The listing builds one solid part. Answer for the finished solid, in the listing's coordinates (mm). A direction names the side the tool comes from. Round coordinates to 2 decimals unless told otherwise and drop trailing zeros. Loops run counter-clockwise (first coordinate to the right, second up) from the corner with the lowest first, then second, coordinate; pieces in that order, holes last. Notation, with made-up numbers: M 1,80.5 L 7,80.5 A13 cw 7,96.5 Z; hole C -4,61.25 d7. An arc over 180 degrees is marked long. Put each result on its own line as item: value. Start each with the question number.
(1) Determine the mould class of faces 4 (the face through (-66, 25.4, -17)), 5 (the face through (-50.651, 22.269, 85.774)), 6 (the face through (-102.283, 22.181, -22.713)) for opening direction X: released by +X, released by -X, zero draft, split by the parting line, or undercut.
(2) Section B-B, the plane z = 0 is taken. Determine the outline of the cut face in (x, y) (3 decimals).
(3) Section A-A, the plane x = 0 is taken. Determine the outline of the cut face in (y, z) (3 decimals).
(4) Which of the six approach directions +Z, -Z, +X, -X, +Y, -Y give full straight-line access (tool end or side, diameter ignored) to faces 1 (the face through (-94.7, 22.3, 0.1)), 2 (the face through (-62, 19.05, 54)), 3 (the face through (73.663, 23.434, -9.672))?
(5) Section D-D, the plane z = -64.5 is taken. Determine the outline of the cut face in (x, y), then the cut area to 3 significant figures.
(6) Flat-ended cylindrical pins translate along their axes: P1, Ø6.5, axis at x = 0, z = -97.25, coming from the -Y side; P2, Ø4, axis at x = -22.5, y = 18, coming from the -Z side; P3, Ø12, axis at x = -42.5, y = 3.5, coming from the -Z side; P4, Ø4, axis at x = 84.22, z = 48.63, coming from the -Y side. Find the tip coordinate at first contact, or state that the pin passes through.
(7) Straight lines are drawn through the part: line 1 (Z direction, x = -16, y = 23.75); line 2 (Z direction, x = 2.5, y = 6.25); line 3 (X direction, y = 4.25, z = -6). For each, find the intervals that lie inside material, in ascending order.
(8) Section C-C, the plane x = -31.5 is taken. Determine the outline of the cut face in (y, z), then the cut area to 3 significant figures.
```python
from build123d import *

# Parameters (mm, degrees)
SKETCH1_R            = 80.518
SKETCH1_R_2          = 67.818
INNER_CYLINDER_DEPTH = 19.05
SKETCH2_R            = 104.775
SKETCH2_R_2          = 67.818
FLANGE_DEPTH         = 6.35
SKETCH4_R            = 81.407
SKETCH4_R_2          = 74.295
GROOVE_DEPTH         = 3.9878
SKETCH5_R            = 2.5527
SCREW_HOLES_DEPTH    = 6.35
CIRPATTERN1_COUNT    = 12


with BuildPart() as part:
    # Sketch1 → Inner Cylinder (new body)
    with BuildSketch(Plane(origin=(0, 0, 0), x_dir=(1, 0, 0), z_dir=(0, 1, 0))):
        with Locations(Location((0, 0, 0), (0, 0, 90))):
            Circle(SKETCH1_R)
        with Locations(Location((0, 0, 0), (0, 0, 90))):
            Circle(SKETCH1_R_2, mode=Mode.SUBTRACT)
    extrude(amount=INNER_CYLINDER_DEPTH)

    # Sketch2 → Flange (add)
    with BuildSketch(Plane(origin=(0, 19.05, 0), x_dir=(1, 0, 0), z_dir=(0, 1, 0))):
        with Locations(Location((0, 0, 0), (0, 0, 270))):
            Circle(SKETCH2_R)
        with Locations(Location((0, 0, 0), (0, 0, 90))):
            Circle(SKETCH2_R_2, mode=Mode.SUBTRACT)
    extrude(amount=FLANGE_DEPTH)

    # Sketch4 → Groove (cut)
    with BuildSketch(Plane(origin=(0, 25.4, 0), x_dir=(1, 0, 0), z_dir=(0, 1, 0))):
        with Locations(Location((0, 0, 0), (0, 0, 270))):
            Circle(SKETCH4_R)
        with Locations(Location((0, 0, 0), (0, 0, 270))):
            Circle(SKETCH4_R_2, mode=Mode.SUBTRACT)
    extrude(amount=-GROOVE_DEPTH, mode=Mode.SUBTRACT)

    # Sketch5 → Screw Holes (cut)
    with BuildSketch(Plane(origin=(0, 25.4, 0), x_dir=(1, 0, 0), z_dir=(0, 1, 0))):
        with Locations(Location((0, -97.25025, 0), (0, 0, 270))):
            Circle(SKETCH5_R)
    screw_holes = extrude(amount=-SCREW_HOLES_DEPTH, mode=Mode.SUBTRACT)

    # CirPattern1: Screw Holes ×12 about axis
    cirpattern1_axis = Axis((0, 0, 0), (0, 1, 0))
    for i in range(1, CIRPATTERN1_COUNT):
        add(screw_holes.rotate(cirpattern1_axis, i * 360 / CIRPATTERN1_COUNT), mode=Mode.SUBTRACT)


solid = part.part
```
Recorded:
1. face 4: zero draft
1. face 5: undercut
1. face 6: split by the parting line
2. outline: M -104.775,19.05 L -99.803,19.05 L -99.803,25.4 L -104.775,25.4 Z; M -94.698,19.05 L -80.518,19.05 L -80.518,0 L -67.818,0 L -67.818,25.4 L -74.295,25.4 L -74.295,21.412 L -81.407,21.412 L -81.407,25.4 L -94.698,25.4 Z; M 67.818,0 L 80.518,0 L 80.518,19.05 L 94.698,19.05 L 94.698,25.4 L 81.407,25.4 L 81.407,21.412 L 74.295,21.412 L 74.295,25.4 L 67.818,25.4 Z; M 99.803,19.05 L 104.775,19.05 L 104.775,25.4 L 99.803,25.4 Z
3. outline: M 0,-80.518 L 19.05,-80.518 L 19.05,-94.698 L 25.4,-94.698 L 25.4,-81.407 L 21.412,-81.407 L 21.412,-74.295 L 25.4,-74.295 L 25.4,-67.818 L 0,-67.818 Z; M 0,67.818 L 25.4,67.818 L 25.4,74.295 L 21.412,74.295 L 21.412,81.407 L 25.4,81.407 L 25.4,94.698 L 19.05,94.698 L 19.05,80.518 L 0,80.518 Z; M 19.05,-104.775 L 25.4,-104.775 L 25.4,-99.803 L 19.05,-99.803 Z; M 19.05,99.803 L 25.4,99.803 L 25.4,104.775 L 19.05,104.775 Z
4. face 1: +Y, -Y
4. face 2: -Y
4. face 3: +Y
5. outline: M -82.57,19.05 L -48.2,19.05 L -48.2,0 L -20.95,0 L -20.95,25.4 L -36.87,25.4 L -36.87,21.41 L -49.67,21.41 L -49.67,25.4 L -82.57,25.4 Z; M 20.95,0 L 48.2,0 L 48.2,19.05 L 82.57,19.05 L 82.57,25.4 L 49.67,25.4 L 49.67,21.41 L 36.87,21.41 L 36.87,25.4 L 20.95,25.4 Z
5. area: 1,720 mm²
6. P1: stops at y = 19.05
6. P2: stops at z = -102.69
6. P3: stops at z = -71.77
6. P4: passes through
7. line 1: z = -103.55 to -79.82, -72.55 to -65.9, 65.9 to 72.55, 79.82 to 103.55
7. line 2: z = -80.48 to -67.77, 67.77 to 80.48
7. line 3: x = -80.29 to -67.55, 67.55 to 80.29
8. outline: M 0,-74.1 L 19.05,-74.1 L 19.05,-99.93 L 25.4,-99.93 L 25.4,-75.07 L 21.41,-75.07 L 21.41,-67.29 L 25.4,-67.29 L 25.4,-60.06 L 0,-60.06 Z; M 0,60.06 L 25.4,60.06 L 25.4,67.29 L 21.41,67.29 L 21.41,75.07 L 25.4,75.07 L 25.4,99.93 L 19.05,99.93 L 19.05,74.1 L 0,74.1 Z
8. area: 979 mm²
